```python
from build123d import *

# Parameters (mm, degrees)
F0_W     = 140
F0_H     = 20
F1_DEPTH = 20
F3_DEPTH = 5


with BuildPart() as f1:
    # F0 (on Front) → F1 (new body)
    with BuildSketch(Plane.XZ):
        with Locations((0, -60)):
            Rectangle(F0_W, F0_H)
        with BuildLine():
            Line((-70, -50), (70, -50))
            Line((70, -50), (25, 55))
            ThreePointArc((25, 55), (18.5187341548, 64.2068689629), (8.8640526043, 70))
            Line((8.8640526043, 70), (-8.8640526043, 70))
            ThreePointArc((-8.8640526043, 70), (-18.5187341548, 64.2068689629), (-25, 55))
            Line((-25, 55), (-70, -50))
        make_face()
        with BuildLine():
            Line((-8.8640526043, 70), (8.8640526043, 70))
            ThreePointArc((8.8640526043, 70), (0, 71.4849039495), (-8.8640526043, 70))
        make_face()
    extrude(amount=F1_DEPTH)

    # F2 (on face) → F3 (cut)
    with BuildSketch(Plane(origin=(0, 0, 0), x_dir=(-1, 0, 0), z_dir=(0, 1, 0))):
        with BuildLine():
            ThreePointArc((11, 51.4849039495), (7.7781745931, 59.2630785426), (0, 62.4849039495))
            ThreePointArc((0, 62.4849039495), (-7.7781745931, 43.7067293565), (11, 51.4849039495))
        make_face()
    extrude(amount=-F3_DEPTH, mode=Mode.SUBTRACT)


solid = f1.part
```
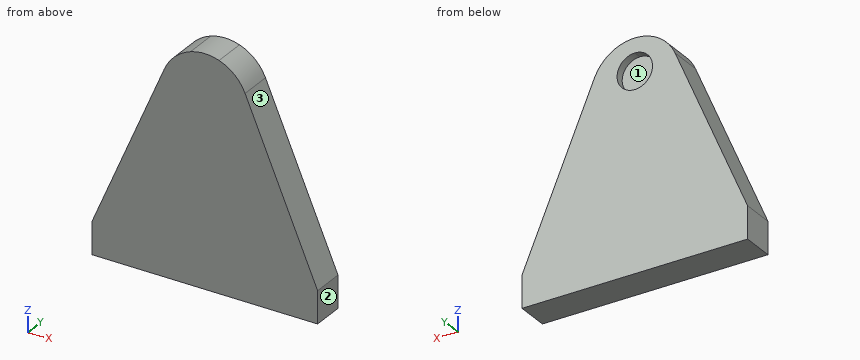
Model file for the job. Use its own axes, mm. Face numbers are marked on the shaded views. Coordinates: 2 decimals unless noted, no trailing zeros. Order: outer loops, then holes, each group sorted by start corner. A loop starts at its lowest first (then second) coordinate and runs counter-clockwise, first axis right, second up. Notation, with made-up numbers: (73, -37) -> (131, -37) arc R27 cw to (131, -16) -> close; hole circle Ø9 at (65.25, 57). An arc over 180 degrees is marked (long way). Return JSON: item names as keys, results as strings.
Item 1: Slice it at D-D (z = 19.5). Write the cut outline in (x, y).
Model answer:
{"outline": "(-40.21, -20) -> (40.21, -20) -> (40.21, 0) -> (-40.21, 0) -> close"}
Item 2: Slice it at A-A (y = -9.5). Write the cut outline in (x, z).
Model answer:
{"outline": "(-70, -70) -> (70, -70) -> (70, -50) -> (25, 55) arc R27.2 ccw to (-25, 55) -> (-70, -50) -> close"}
Item 3: Slice it at B-B (z = 46). Write the cut outline in (x, y), then the cut area to 3 significant figures.
Model answer:
{"outline": "(-28.86, -20) -> (28.86, -20) -> (28.86, 0) -> (9.53, 0) -> (9.53, -5) -> (-9.53, -5) -> (-9.53, 0) -> (-28.86, 0) -> close", "area": "1,060 mm²"}
Item 4: Wall check: line 1 along Z through (x, y) = (0, -3.5); line 2 along Y through (x, z) = (4, 60); line 3 along Z through (x, y) = (4.5, -3.25). Give the ranges that are in metal, low to high. Write a range as from..to.
Model answer:
{"line 1": "z = -70..40.48, 62.48..71.48", "line 2": "y = -20..-5", "line 3": "z = -70..41.45, 61.52..71.11"}
Item 5: Mould opens along Z. For the marked faces 1, 2 and 3 say: pulls with the +Z half, pulls with the -Z half, needs draft (parallel to the pull), parting line crosses it, or undercut.
Model answer:
{"face 1": "undercut", "face 2": "needs draft", "face 3": "pulls with the +Z half"}
Item 6: Pin check, flat tips, straight feed: P1, Ø6, axis at y = -14.5, z = -6, coming from the +X side; P2, Ø1, axis at y = -10.5, z = 46, coming from the +X side; P3, Ø1, axis at y = -16.5, z = 26, coming from the -X side. Stop position of each tip, or through.
Model answer:
{"P1": "stops at x = 52.43", "P2": "stops at x = 29.07", "P3": "stops at x = -37.64"}
Item 7: Slice it at C-C (x = 53). Write the cut outline in (y, z), then the cut area to 3 significant figures.
Model answer:
{"outline": "(-20, -70) -> (0, -70) -> (0, -10.33) -> (-20, -10.33) -> close", "area": "1,190 mm²"}
